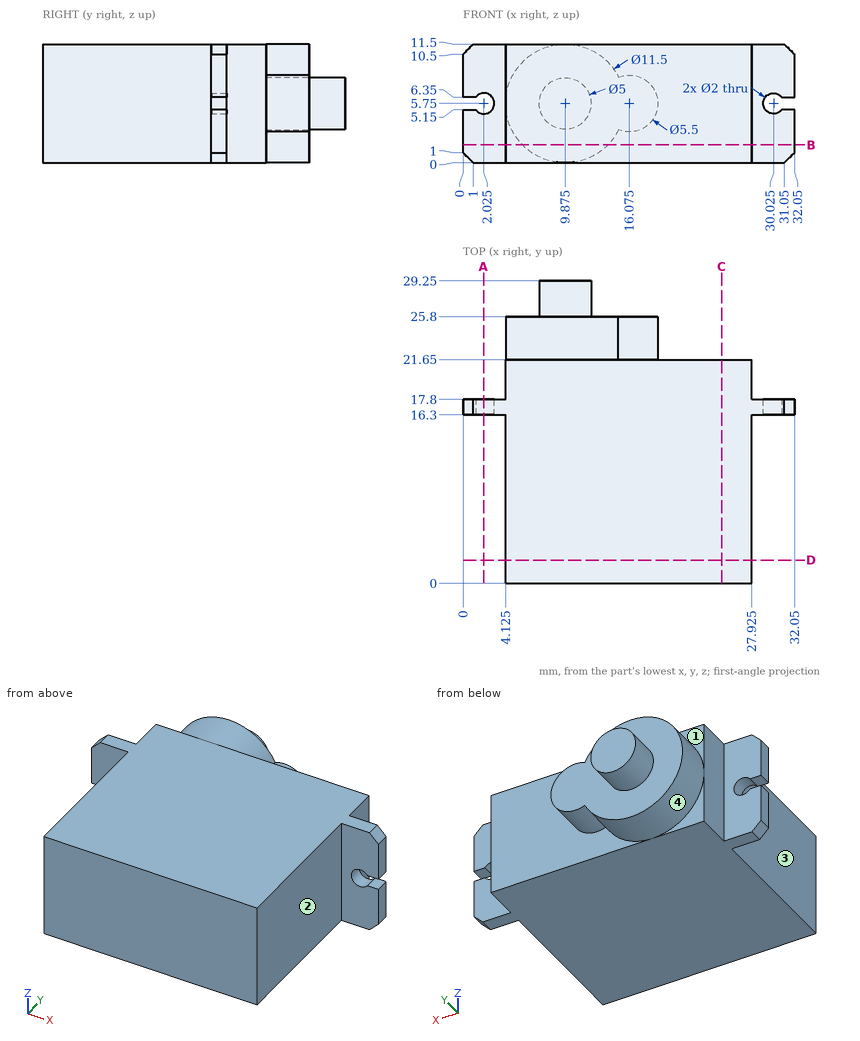
Job drawing, mm, ordinate dimensions from the low corner. One solid piece. A direction names the side the tool comes from. Round coordinates to 2 decimals unless told otherwise and drop trailing zeros. Write each loop counter-clockwise with the first axis right and the second up, starting at its lowest first coordinate (ties: lowest second). Pieces come first, ordered by that corner, then holes.
1) Band-saw the part on B-B, the plane z = 1.75. List the corners of the cut face in (x, y) (3 decimals).
2) Drill centre lines: probe 1 along X at (y, z) = (16.8, 5.75) (3 decimals); probe 2 along Y at (x, z) = (28.5, 7); probe 3 along Y at (x, z) = (27, 3.25). Where is each one in solid material? Low to high.
3) Band-saw the part on D-D, the plane y = 2.25. List the corners of the cut face in (x, z) (3 decimals).
4) 3-axis set-ups, long thin cutter, end or side, ignore diameter. For the marked faces 1, 2, 3 and 4: which of +Z, -Z, +X, -X, +Y, -Y reach the whole face in a straight line?
5) Pin check, flat tips, straight feed: pin 1 (6 mm diameter, centred on y = 12, z = 6, fed in from +X) (3 decimals); pin 2 (3.5 mm diameter, centred on x = 2, z = 6.5, fed in from +Y); pin 3 (3.5 mm diameter, centred on x = 21, z = 7, fed in from +Y). Stop position of each tip, or through.
6) Band-saw the part on A-A, the plane x = 2. List the corners of the cut face in (y, z), and give its area (3 significant figures).
7) Band-saw the part on C-C, the plane x = 25. List the corners of the cut face in (y, z).
Ans:
1. outline: (0, 16.3) - (4.125, 16.3) - (4.125, 0) - (27.925, 0) - (27.925, 16.3) - (32.05, 16.3) - (32.05, 17.8) - (27.925, 17.8) - (27.925, 21.65) - (14.006, 21.65) - (14.006, 25.8) - (5.744, 25.8) - (5.744, 21.65) - (4.125, 21.65) - (4.125, 17.8) - (0, 17.8) - close
2. probe 1: x = 3.025 to 29.025
2. probe 2: y = 16.3 to 17.8
2. probe 3: y = 0 to 21.65
3. outline: (4.125, 0) - (27.925, 0) - (27.925, 11.5) - (4.125, 11.5) - close
4. face 1: +Z, -X, +Y
4. face 2: +Z, -Z, +X, -Y
4. face 3: +Z, -Z, -X, -Y
4. face 4: +Y
5. pin 1: stops at x = 27.925
5. pin 2: stops at y = 17.8
5. pin 3: stops at y = 21.65
6. outline: (16.3, 0) - (17.8, 0) - (17.8, 4.75) - (16.3, 4.75) - close; (16.3, 6.75) - (17.8, 6.75) - (17.8, 11.5) - (16.3, 11.5) - close
6. area: 14.3 mm2
7. outline: (0, 0) - (21.65, 0) - (21.65, 11.5) - (0, 11.5) - close
